For this review, take the finished solid that the model builds, in its own axes (mm). A direction names the side the tool comes from. Give positions to 0.01 mm unless a question says otherwise; leave off trailing zeros. Loops run counter-clockwise (first coordinate to the right, second up) from the corner with the lowest first, then second, coordinate; pieces in that order, holes last. Notation, with made-up numbers: (82.5, 76) - (131.5, 76) arc R17 cw to (131.5, 88) - close; hole circle Ø1 at (87, 15.5). An arc over 180 degrees is marked (long way). Use CSV: the item, a comma, the result in double quotes. Start each with the question number.
1. Take a section at D-D on x = 4. Give the boundary of the cut face in (y, z), plus the area to 3 significant figures.
2. Mouldability with a two-part tool opening along Z and no side actions: class faces 1 (the cylindrical face through (-0.28, 1.77, -38.79)), 2 (the flat face through (0, 6, -2)), 3 (the cylindrical face through (0, 1, 5)) as pulls with the +Z half, pulls with the -Z half, needs draft (parallel to the pull), parting line crosses it, or undercut.
3. Take a section at B-B on y = 0.7. Give the boundary of the cut face in (x, z), plus the area to 3 significant figures.
4. For faces 4 (the flat face through (-5, 1, -17)), 5 (the flat face through (5, 1, -17)), 6 (the flat face through (0.4, 3.2, -35)), 7 (the flat face through (-1.3, 3.5, -39)), list the 3-axis set-ups (+Z, -Z, +X, -X, +Y, -Y) from which the entire face can be reached by the end or side of a thin tool; tool diameter is ignored.
5. Wall thickness on line 1 (Z direction, x = 0, y = 1.5); line 2 (Z direction, x = 0, y = 3.6); line 3 (Z direction, x = -1, y = 1.3): over which ranges is each line inside the solid? List them lowest first.
6. Take a section at A-A on z = -40.5. Give the boundary of the cut face in (x, y).
7. For pin 1 (3 mm diameter, centred on x = 0, z = 0, fed in from -Y) (3 decimals); pin 2 (3.5 mm diameter, centred on y = 1, z = -11, fed in from -X); pin 3 (2.5 mm diameter, centred on y = 2, z = -18.5, fed in from +X); pin 4 (2 mm diameter, centred on x = 0.5, z = -11.5, fed in from +Y), all flat-tipped, find the tip position at first contact; note any pin that passes through.
8. Take a section at C-C on x = 0.1. Give the boundary of the cut face in (y, z), plus the area to 3 significant figures.
Autodesk Inventor part; units mm, degrees
ref_plane "YZ Plane" through (0, 0, 0) normal (1, 0, 0) x (0, 1, 0)
ref_plane "XZ Plane" through (0, 0, 0) normal (0, 1, 0) x (-1, 0, 0)
ref_plane "XY Plane" through (0, 0, 0) normal (0, 0, 1) x (1, 0, 0)
sketch "Sketch1" plane through (0, 0, 0) normal (0, 1, 0) x (-1, 0, 0)
  circle A0 centre (0, 0) radius 1.75
  arc A1 (5, 0) -> (-5, 0) centre (0, 0) ccw
  circle A2 centre (0, 0) radius 3
  line L0 (5, 0) -> (5, -5)
  line L1 (5, -5) -> (-5, -5)
  line L2 (-5, 0) -> (-5, -5)
  dimension "d0" = 3.5
  dimension "d1" = 10
  dimension "d2" = 6
extrude "Extrusion1" add sketch "Sketch1" along normal blind 3 contours L0 L1 L2 A1
extrude "bearing-distance-holder" add sketch "Sketch1" along normal blind 6 contours A2
sketch "Sketch2" plane through (5, 0, -5) normal (0, 0, -1) x (-1, 0, 0)
  line L0 (0, 0) -> (10, 0)
  line L1 (10, 0) -> (10, 3)
  line L2 (0, 3) -> (10, 3)
  line L3 (0, 0) -> (0, 3)
  point P0 (5, 0)
extrude "L" add sketch "Sketch2" along normal blind 40
sketch "Sketch6" plane through (5, 0, -45) normal (0, 0, -1) x (-1, 0, 0)
  line L0 (10.3, 3.5) -> (-0.3, 3.5)
  line L1 (-0.3, 3.5) -> (-0.3, 0)
  line L2 (-0.3, 0) -> (10.3, 0)
  line L3 (10.3, 0) -> (10.3, 3.5)
  line L4 (10, 0) -> (10, 3)
  line L5 (0, 0) -> (10, 0)
  line L6 (10, 3) -> (0, 3)
  line L7 (0, 3) -> (0, 0)
  point P0 (5, 0)
  dimension "d20" = 0.3
  dimension "d21" = 0
  dimension "d22" = 0.5
  dimension "d23" = 0.3
extrude "Extrusion7" add sketch "Sketch6" against normal blind 10 contours L3 L2 L4 L6 L7 L1 L0
sketch "Sketch5" plane through (0.1, 3.5, 0) normal (0, 1, 0) x (1, 0, 0)
  circle A0 centre (0, 40.5) radius 1.75
  line L0 (-5, 45) -> (5, 45)
  point P0 (-0.1, 0)
  dimension "d16" = 4.5
  dimension "d17" = 3.5
extrude "Extrusion8" cut sketch "Sketch5" along normal mid plane 10
properties part number "connecting-rod-40"
Check result:
1,outline,"(0, -45) - (3.5, -45) - (3.5, -35) - (3, -35) - (3, 3) - (0, 3) - close"
1,area,"149 mm²"
2,face 1,"undercut"
2,face 2,"needs draft"
2,face 3,"pulls with the +Z half"
3,outline,"(-5.3, -45) - (5.3, -45) - (5.3, -35) - (5, -35) - (5, 0) arc R5 ccw to (-5, 0) - (-5, -35) - (-5.3, -35) - close; hole circle Ø3.5 at (0, 0); hole circle Ø3.5 at (0.1, -40.5)"
3,area,"476 mm²"
4,face 4,"+Z, -X, +Y, -Y"
4,face 5,"+Z, +X, +Y, -Y"
4,face 6,"+Y"
4,face 7,"-Z, +X, -X, +Y"
5,line 1,"z = -45 to -42.25, -38.75 to -1.75, 1.75 to 5"
5,line 2,"z = -3 to -1.75, 1.75 to 3"
5,line 3,"z = -45 to -41.86, -39.14 to -1.44, 1.44 to 4.9"
6,outline,"(-5.3, 0) - (-1.65, 0) - (-1.65, 3.5) - (-5.3, 3.5) - close; (1.85, 0) - (5.3, 0) - (5.3, 3.5) - (1.85, 3.5) - close"
7,pin 1,"passes through"
7,pin 2,"stops at x = -5"
7,pin 3,"stops at x = 5"
7,pin 4,"stops at y = 3"
8,outline,"(0, -45) - (3.5, -45) - (3.5, -42.25) - (0, -42.25) - close; (0, -38.75) - (3.5, -38.75) - (3.5, -35) - (3, -35) - (3, -3) - (6, -3) - (6, -1.75) - (0, -1.75) - close; (0, 1.75) - (6, 1.75) - (6, 3) - (3, 3) - (3, 5) - (0, 5) - close"
8,area,"140 mm²"
